Could you check a few things on this model? Use its own coordinates, in mm. Face numbers are marked on the shaded views. A direction names the side the tool comes from. Coordinates: 2 decimals unless noted, no trailing zeros. Write each loop counter-clockwise with the first axis right and the second up, starting at its lowest first coordinate (ties: lowest second). Pieces come first, ordered by that corner, then holes.
Item 1: Which directions (+Z, -Z, +X, -X, +Y, -Y) give clear straight access to the entire face, cutting with the end or side of a thin tool? Please do the marked faces 4 and 5.
Item 2: I want a section at D-D on z = -20. Please give me the cut outline in (x, y).
Item 3: For P1, Ø5.5, axis at x = -24.5, y = -25.5, coming from the +Z side; P2, Ø10, axis at x = -28.5, y = -12.5, coming from the +Z side; P3, Ø8, axis at x = 23.5, z = -10.5, coming from the -Y side; P4, Ø10.5, axis at y = -29, z = 1.5, coming from the -X side, each with a flat end and sliding along its axis, tell me the tip position at first contact or that it passes through.
Item 4: If I drill on probe 1 along X at (y, z) = (-18.5, -5); probe 2 along Y at (x, z) = (21, 8.5); probe 3 along Z at (x, y) = (-52, -23), over which ranges is the centre line in solid material (lowest first)?
Item 5: Thinking about a two-plate mould opening in X: for the marked faces 1, 2 and 3, which applies, +X half, -X half, draft (parallel to the pull), parting line (faces both ways), or undercut?
Item 6: I want a section at B-B on z = -6.5. Please give me the cut outline in (x, y).
Item 7: I want a section at A-A on x = 46. Please give me the cut outline in (y, z).
from build123d import *

# Parameters (mm, degrees)
F0_R     = 10.367684
F1_DEPTH = 25.4
F2_DEPTH = 45.974


with BuildPart() as f1:
    # F0 (on Front) → F1 (new body)
    with BuildSketch(Plane.XZ):
        with BuildLine():
            Line((-35.898636, 24.557869), (-41.97927, 25.158544))
            ThreePointArc((-41.97927, 25.158544), (-66.554008, 0.545011), (-43.068193, -25.109624))
            Line((-43.068193, -25.109624), (-34.926978, -24.320042))
            ThreePointArc((-34.926978, -24.320042), (-21.443966, -15.338432), (-16.229235, 0))
            ThreePointArc((-16.229235, 0), (-21.752764, 15.731928), (-35.898636, 24.557869))
        make_face()
        with BuildLine():
            ThreePointArc((-56.674072, 4.680658), (-41.394573, 15.980353), (-26.115073, 4.680658))
            Line((-26.115073, 4.680658), (-20.916691, 4.680658))
            Line((-20.916691, 4.680658), (-20.916691, -4.671074))
            Line((-20.916691, -4.671074), (-26.112141, -4.671074))
            ThreePointArc((-26.112141, -4.671074), (-41.394573, -15.980353), (-56.677005, -4.671074))
            ThreePointArc((-56.677005, -4.671074), (-57.374925, 0), (-56.677005, 4.671074))
            Line((-56.677005, 4.671074), (-56.677005, 4.680658))
            Line((-56.677005, 4.680658), (-56.674072, 4.680658))
        make_face(mode=Mode.SUBTRACT)
        with BuildLine():
            ThreePointArc((-35.898636, 24.557869), (-38.920654, 25.043441), (-41.97927, 25.158544))
            Line((-41.97927, 25.158544), (-35.898636, 24.557869))
        make_face()
        with BuildLine():
            Line((-34.926978, -24.320042), (-43.068193, -25.109624))
            ThreePointArc((-43.068193, -25.109624), (-38.965291, -25.047811), (-34.926978, -24.320042))
        make_face()
        with BuildLine():
            Line((43.919244, 16.673053), (-35.898636, 24.557869))
            ThreePointArc((-35.898636, 24.557869), (-21.752764, 15.731928), (-16.229235, 0))
            ThreePointArc((-16.229235, 0), (-21.443966, -15.338432), (-34.926978, -24.320042))
            Line((-34.926978, -24.320042), (43.889526, -16.675962))
            ThreePointArc((43.889526, -16.675962), (25.517994, 0.01493), (43.919244, 16.673053))
        make_face()
        with BuildLine():
            ThreePointArc((59.026403, 0), (54.68788, 11.249633), (43.919244, 16.673053))
            ThreePointArc((43.919244, 16.673053), (25.517994, 0.01493), (43.889526, -16.675962))
            ThreePointArc((43.889526, -16.675962), (54.677851, -11.260692), (59.026403, 0))
        make_face()
        with Locations((42.272195, 0)):
            Circle(F0_R, mode=Mode.SUBTRACT)
    extrude(amount=F1_DEPTH)

    # F0 (on Front) → F2 (join)
    with BuildSketch(Plane.XZ):
        with BuildLine():
            Line((-35.898636, 24.557869), (-41.97927, 25.158544))
            ThreePointArc((-41.97927, 25.158544), (-66.554008, 0.545011), (-43.068193, -25.109624))
            Line((-43.068193, -25.109624), (-34.926978, -24.320042))
            ThreePointArc((-34.926978, -24.320042), (-21.443966, -15.338432), (-16.229235, 0))
            ThreePointArc((-16.229235, 0), (-21.752764, 15.731928), (-35.898636, 24.557869))
        make_face()
        with BuildLine():
            ThreePointArc((-56.674072, 4.680658), (-41.394573, 15.980353), (-26.115073, 4.680658))
            Line((-26.115073, 4.680658), (-20.916691, 4.680658))
            Line((-20.916691, 4.680658), (-20.916691, -4.671074))
            Line((-20.916691, -4.671074), (-26.112141, -4.671074))
            ThreePointArc((-26.112141, -4.671074), (-41.394573, -15.980353), (-56.677005, -4.671074))
            ThreePointArc((-56.677005, -4.671074), (-57.374925, 0), (-56.677005, 4.671074))
            Line((-56.677005, 4.671074), (-56.677005, 4.680658))
            Line((-56.677005, 4.680658), (-56.674072, 4.680658))
        make_face(mode=Mode.SUBTRACT)
    extrude(amount=F2_DEPTH)


solid = f1.part
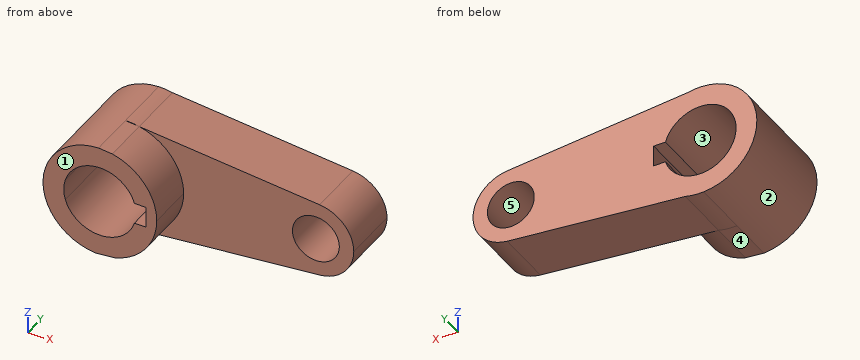
Response values:
1. face 4: -Z, +X, -Y
1. face 5: +Y, -Y
2. outline: (-56.67, -45.97) - (-26.12, -45.97) - (-26.12, -25.4) - (9.62, -25.4) - (9.62, 0) - (-56.67, 0) - close
3. P1: stops at z = 23.7
3. P2: stops at z = 24.32
3. P3: stops at y = -25.4
3. P4: stops at x = -66.56
4. probe 1: x = -66.06 to -56.57, -26.22 to 33.19, 51.35 to 58.26
4. probe 2: y = -25.4 to 0
4. probe 3: z = -22.82 to -11.95, 11.95 to 22.82
5. face 1: draft
5. face 2: -X half
5. face 3: undercut
6. outline: (-65.71, -45.97) - (-55.99, -45.97) - (-55.99, 0) - (-65.71, 0) - close; (-26.8, -45.97) - (-17.08, -45.97) - (-17.08, -25.4) - (34.2, -25.4) - (34.2, 0) - (-26.8, 0) - close; (50.35, -25.4) - (57.71, -25.4) - (57.71, 0) - (50.35, 0) - close
7. outline: (-25.4, -16.33) - (0, -16.33) - (0, -9.67) - (-25.4, -9.67) - close; (-25.4, 9.67) - (0, 9.67) - (0, 16.33) - (-25.4, 16.33) - close
